Input: part model. Units: mm. Frame: model coordinates. A direction names the side the tool comes from. Give positions to 0.01 mm unless a question says otherwise; leave off trailing zeros. Order: outer loops, then holes, each group sorted by start corner. A loop starts at its lowest first (then second) coordinate and runs counter-clockwise, first axis right, second up. Notation, with made-up numbers: (85.25, 19) - (98.25, 19) arc R28 ccw to (98.25, 53) - close; hole circle Ø10 at (31.25, -20.75). An arc over 180 degrees is marked (long way). Use a Markdown table: item, result.
from build123d import *

# Parameters (mm, degrees)
SKETCH1_W           = 35
SKETCH1_H           = 20
SKETCH1_R           = 1.65
BOSS_EXTRUDE1_DEPTH = 5
SKETCH3_W           = 18
SKETCH3_H           = 4
BOSS_EXTRUDE2_DEPTH = 25
CUT_EXTRUDE1_REACH  = 40.239
SKETCH4_R           = 2.15
SKETCH5_R           = 3
CUT_EXTRUDE2_DEPTH  = 2
CHAMFER1_SIZE2      = 9.237604307
CHAMFER1_SIZE       = 16


with BuildPart() as part:
    # Sketch1 → Boss-Extrude1 (new body)
    with BuildSketch(Plane(origin=(0, 0, 0), x_dir=(1, 0, 0), z_dir=(0, 1, 0))):
        Rectangle(SKETCH1_W, SKETCH1_H)
        with Locations(Location((-12.5, 0, 0), (0, 0, 270))):
            Circle(SKETCH1_R, mode=Mode.SUBTRACT)
        with Locations(Location((12.5, 0, 0), (0, 0, 90))):
            Circle(SKETCH1_R, mode=Mode.SUBTRACT)
    extrude(amount=BOSS_EXTRUDE1_DEPTH)

    # Sketch3 → Boss-Extrude2 (add)
    with BuildSketch(Plane(origin=(0, 5, 0), x_dir=(1, 0, 0), z_dir=(0, 1, 0))):
        with Locations((0, 8)):
            Rectangle(SKETCH3_W, SKETCH3_H)
    extrude(amount=BOSS_EXTRUDE2_DEPTH)

    # Sketch4 → Cut-Extrude1 (cut, up to next)
    with BuildSketch(Plane.XY.offset(-6), mode=Mode.PRIVATE) as cut_extrude1_sk1:
        with Locations((-4, 23)):
            Circle(SKETCH4_R)
    cut_extrude1_tool1 = extrude(cut_extrude1_sk1.sketch, amount=-CUT_EXTRUDE1_REACH, mode=Mode.PRIVATE) & part.part
    # Sketch4 → Cut-Extrude1 (cut, up to next)
    with BuildSketch(Plane.XY.offset(-6), mode=Mode.PRIVATE) as cut_extrude1_sk2:
        with Locations((4, 26.5)):
            Circle(SKETCH4_R)
    cut_extrude1_tool2 = extrude(cut_extrude1_sk2.sketch, amount=-CUT_EXTRUDE1_REACH, mode=Mode.PRIVATE) & part.part
    # Sketch4 → Cut-Extrude1 (cut, up to next)
    with BuildSketch(Plane.XY.offset(-6), mode=Mode.PRIVATE) as cut_extrude1_sk3:
        with Locations((4, 19.5)):
            Circle(SKETCH4_R)
    cut_extrude1_tool3 = extrude(cut_extrude1_sk3.sketch, amount=-CUT_EXTRUDE1_REACH, mode=Mode.PRIVATE) & part.part
    add(cut_extrude1_tool1.solids().sort_by_distance((-4, 23, -6))[0], mode=Mode.SUBTRACT)
    add(cut_extrude1_tool2.solids().sort_by_distance((4, 26.5, -6))[0], mode=Mode.SUBTRACT)
    add(cut_extrude1_tool3.solids().sort_by_distance((4, 19.5, -6))[0], mode=Mode.SUBTRACT)

    # Sketch5 → Cut-Extrude2 (cut)
    with BuildSketch(Plane(origin=(0, 5, 0), x_dir=(1, 0, 0), z_dir=(0, 1, 0))):
        with Locations(Location((-12.5, 0, 0), (0, 0, 270))):
            Circle(SKETCH5_R)
        with Locations(Location((12.5, 0, 0), (0, 0, 90))):
            Circle(SKETCH5_R)
    extrude(amount=-CUT_EXTRUDE2_DEPTH, mode=Mode.SUBTRACT)

    # Chamfer1
    chamfer1_edges = [part.edges().sort_by_distance(p)[0] for p in [
        (0, 5, -6),
    ]]
    chamfer1_side = [part.faces().sort_by_distance(p)[0] for p in [
        (0, 5, -5.815247914),
    ]]
    chamfer(chamfer1_edges, length=CHAMFER1_SIZE - 0.0001, length2=CHAMFER1_SIZE2 - 0.0001, reference=chamfer1_side[0])  # a hair under: the kernel refuses the full size


solid = part.part
1. Set-up query: faces 1 (the face through (14.1, 1.5, 0.4)), 2 (the face through (0, 22, -6)), 3 (the face through (15.162, 4.014, -1.384)), 4 (the face through (9, 12, -4)). Return all of +Z, -Z, +X, -X, +Y, -Y with unobstructed straight access to the full face (end or side cutting, diameter ignored); none if empty.
Response:
| item | result |
|---|---|
| face 1 | +Y, -Y |
| face 2 | +Z, +X, -X, +Y |
| face 3 | +Y |
| face 4 | +Z, -Z, +X, +Y |
2. Mould query, pull axis X, two halves, no side actions, for faces 5 (the face through (-4.47, 20.9, -7.97)), 6 (the face through (-9, 12, -4)), 7 (the face through (0, 2, 10)). Classes: pulls with the +X half, pulls with the -X half, needs draft (parallel to the pull), parting line crosses it, or undercut.
Response:
| item | result |
|---|---|
| face 5 | undercut |
| face 6 | pulls with the -X half |
| face 7 | needs draft |
3. Section query A-A (x = 4). State how many separate pieces and enclosed holes the cut face has, then the cut area to 4 significant figures.
Response:
| item | result |
|---|---|
| separate pieces | 3 |
| enclosed holes | 0 |
| area | 239.5 mm^2 |
4. Material intervals for line 1 along X through (y, z) = (3.9, 0); line 2 along Z through (x, y) = (-12.5, 1.4); line 3 along X through (y, z) = (12.5, -6), sorted ascending.
Response:
| item | result |
|---|---|
| line 1 | x = -17.5 to -15.5, -9.5 to 9.5, 15.5 to 17.5 |
| line 2 | z = -10 to -1.65, 1.65 to 10 |
| line 3 | x = -9 to 9 |
5. Section query D-D (z = 0). Return loops of the section in (x, y).
Response:
| item | result |
|---|---|
| outline | (-17.5, 0) - (-14.15, 0) - (-14.15, 3) - (-15.5, 3) - (-15.5, 5) - (-17.5, 5) - close; (-10.85, 0) - (10.85, 0) - (10.85, 3) - (9.5, 3) - (9.5, 5) - (9, 5) - (9, 10.77) - (-9, 10.77) - (-9, 5) - (-9.5, 5) - (-9.5, 3) - (-10.85, 3) - close; (14.15, 0) - (17.5, 0) - (17.5, 5) - (15.5, 5) - (15.5, 3) - (14.15, 3) - close |
6. Pin query (flat end, axial travel): pin 1 (6 mm diameter, centred on x = -3, z = 2, fed in from +Y); pin 2 (12 mm diameter, centred on x = -1, z = -5, fed in from -Y); pin 3 (5 mm diameter, centred on x = 11, z = -1, fed in from +Y); pin 4 (4.5 mm diameter, centred on x = -1, y = 24, fed in from +Z). Return the tip coordinate at first contact, or that it passes through.
Response:
| item | result |
|---|---|
| pin 1 | stops at y = 11.35 |
| pin 2 | stops at y = 0 |
| pin 3 | stops at y = 12.22 |
| pin 4 | stops at z = -6 |
7. Section query B-B (x = 12.5). Return loops of the section in (y, z).
Response:
| item | result |
|---|---|
| outline | (0, -10) - (5, -10) - (5, -3) - (3, -3) - (3, -1.65) - (0, -1.65) - close; (0, 1.65) - (3, 1.65) - (3, 3) - (5, 3) - (5, 10) - (0, 10) - close |
8. Section query C-C (y = 19.5). Return loops of the section in (x, z), then the cut area to 3 significant figures.
Response:
| item | result |
|---|---|
| outline | (-9, -10) - (1.85, -10) - (1.85, -6) - (-9, -6) - close; (6.15, -10) - (9, -10) - (9, -6) - (6.15, -6) - close |
| area | 54.8 mm^2 |
